Build history of the part. All positions in model axes, mm. A direction names the side the tool comes from. Give positions to 0.01 mm unless a question says otherwise; leave off trailing zeros. Order: outer loops, then holes, each group sorted by start corner. A loop starts at its lowest first (then second) coordinate and runs counter-clockwise, first axis right, second up. Notation, with made-up numbers: (-1.5, 57) - (26.5, 57) arc R21 cw to (26.5, 91) - close; hole circle Ø10 at (22, -12). An arc over 180 degrees is marked (long way). Write each question's results on one line, items separated by ' | '. Start each with the question number.
from build123d import *

# Parameters (mm, degrees)
SKETCH_1_R          = 9
SKETCH_1_R_2        = 2.5
EXTRUDE_1_DEPTH     = 1.5
SKETCH_2_R          = 2.5
EXTRUDE_2_DEPTH     = 7.5
SKETCH_3_R          = 9
SKETCH_3_R_2        = 2.5
EXTRUDE_3_DEPTH     = 9
CHAMFER_2_SIZE      = 0.2
SKETCH_4_R          = 1.75
CUT_EXTRUDE_1_DEPTH = 10
SKETCH_5_R          = 1.75
CUT_EXTRUDE_2_DEPTH = 10


with BuildPart() as part:
    # 草图1 → 凸台-拉伸1 (new body)
    with BuildSketch(Plane.XY):
        Circle(SKETCH_1_R)
        Circle(SKETCH_1_R_2, mode=Mode.SUBTRACT)
    extrude(amount=EXTRUDE_1_DEPTH)

    # 草图2 → 凸台-拉伸2 (add)
    with BuildSketch(Plane.XY.offset(1.5)):
        with BuildLine():
            Line((-0.415, 5.98563071), (-0.415, 4.982747736))
            ThreePointArc((-0.415, 4.982747736), (-0.782172325, 4.938441703), (-1.145065275, 4.867116756))
            Line((-1.145065275, 4.867116756), (-1.454973157, 5.820915144))
            Line((-1.454973157, 5.820915144), (-2.244350066, 5.564431038))
            Line((-2.244350066, 5.564431038), (-1.934442183, 4.610632651))
            ThreePointArc((-1.934442183, 4.610632651), (-2.269952499, 4.455032621), (-2.593043582, 4.275058477))
            Line((-2.593043582, 4.275058477), (-3.182523405, 5.086407846))
            Line((-3.182523405, 5.086407846), (-3.85400751, 4.598546087))
            Line((-3.85400751, 4.598546087), (-3.264527688, 3.787196717))
            ThreePointArc((-3.264527688, 3.787196717), (-3.535533906, 3.535533906), (-3.787196717, 3.264527688))
            Line((-3.787196717, 3.264527688), (-4.598546087, 3.85400751))
            Line((-4.598546087, 3.85400751), (-5.086407846, 3.182523405))
            Line((-5.086407846, 3.182523405), (-4.275058477, 2.593043582))
            ThreePointArc((-4.275058477, 2.593043582), (-4.455032621, 2.269952499), (-4.610632651, 1.934442183))
            Line((-4.610632651, 1.934442183), (-5.564431038, 2.244350066))
            Line((-5.564431038, 2.244350066), (-5.820915144, 1.454973157))
            Line((-5.820915144, 1.454973157), (-4.867116756, 1.145065275))
            ThreePointArc((-4.867116756, 1.145065275), (-4.938441703, 0.782172325), (-4.982747736, 0.415))
            Line((-4.982747736, 0.415), (-5.98563071, 0.415))
            Line((-5.98563071, 0.415), (-5.98563071, -0.415))
            Line((-5.98563071, -0.415), (-4.982747736, -0.415))
            ThreePointArc((-4.982747736, -0.415), (-4.938441703, -0.782172325), (-4.867116756, -1.145065275))
            Line((-4.867116756, -1.145065275), (-5.820915144, -1.454973157))
            Line((-5.820915144, -1.454973157), (-5.564431038, -2.244350066))
            Line((-5.564431038, -2.244350066), (-4.610632651, -1.934442183))
            ThreePointArc((-4.610632651, -1.934442183), (-4.455032621, -2.269952499), (-4.275058477, -2.593043582))
            Line((-4.275058477, -2.593043582), (-5.086407846, -3.182523405))
            Line((-5.086407846, -3.182523405), (-4.598546087, -3.85400751))
            Line((-4.598546087, -3.85400751), (-3.787196717, -3.264527688))
            ThreePointArc((-3.787196717, -3.264527688), (-3.535533906, -3.535533906), (-3.264527688, -3.787196717))
            Line((-3.264527688, -3.787196717), (-3.85400751, -4.598546087))
            Line((-3.85400751, -4.598546087), (-3.182523405, -5.086407846))
            Line((-3.182523405, -5.086407846), (-2.593043582, -4.275058477))
            ThreePointArc((-2.593043582, -4.275058477), (-2.269952499, -4.455032621), (-1.934442183, -4.610632651))
            Line((-1.934442183, -4.610632651), (-2.244350066, -5.564431038))
            Line((-2.244350066, -5.564431038), (-1.454973157, -5.820915144))
            Line((-1.454973157, -5.820915144), (-1.145065275, -4.867116756))
            ThreePointArc((-1.145065275, -4.867116756), (-0.782172325, -4.938441703), (-0.415, -4.982747736))
            Line((-0.415, -4.982747736), (-0.415, -5.98563071))
            Line((-0.415, -5.98563071), (0.415, -5.98563071))
            Line((0.415, -5.98563071), (0.415, -4.982747736))
            ThreePointArc((0.415, -4.982747736), (0.782172325, -4.938441703), (1.145065275, -4.867116756))
            Line((1.145065275, -4.867116756), (1.454973157, -5.820915144))
            Line((1.454973157, -5.820915144), (2.244350066, -5.564431038))
            Line((2.244350066, -5.564431038), (1.934442183, -4.610632651))
            ThreePointArc((1.934442183, -4.610632651), (2.269952499, -4.455032621), (2.593043582, -4.275058477))
            Line((2.593043582, -4.275058477), (3.182523405, -5.086407846))
            Line((3.182523405, -5.086407846), (3.85400751, -4.598546087))
            Line((3.85400751, -4.598546087), (3.264527688, -3.787196717))
            ThreePointArc((3.264527688, -3.787196717), (3.535533906, -3.535533906), (3.787196717, -3.264527688))
            Line((3.787196717, -3.264527688), (4.598546087, -3.85400751))
            Line((4.598546087, -3.85400751), (5.086407846, -3.182523405))
            Line((5.086407846, -3.182523405), (4.275058477, -2.593043582))
            ThreePointArc((4.275058477, -2.593043582), (4.455032621, -2.269952499), (4.610632651, -1.934442183))
            Line((4.610632651, -1.934442183), (5.564431038, -2.244350066))
            Line((5.564431038, -2.244350066), (5.820915144, -1.454973157))
            Line((5.820915144, -1.454973157), (4.867116756, -1.145065275))
            ThreePointArc((4.867116756, -1.145065275), (4.938441703, -0.782172325), (4.982747736, -0.415))
            Line((4.982747736, -0.415), (5.98563071, -0.415))
            Line((5.98563071, -0.415), (5.98563071, 0.415))
            Line((5.98563071, 0.415), (4.982747736, 0.415))
            ThreePointArc((4.982747736, 0.415), (4.938441703, 0.782172325), (4.867116756, 1.145065275))
            Line((4.867116756, 1.145065275), (5.820915144, 1.454973157))
            Line((5.820915144, 1.454973157), (5.564431038, 2.244350066))
            Line((5.564431038, 2.244350066), (4.610632651, 1.934442183))
            ThreePointArc((4.610632651, 1.934442183), (4.455032621, 2.269952499), (4.275058477, 2.593043582))
            Line((4.275058477, 2.593043582), (5.086407846, 3.182523405))
            Line((5.086407846, 3.182523405), (4.598546087, 3.85400751))
            Line((4.598546087, 3.85400751), (3.787196717, 3.264527688))
            ThreePointArc((3.787196717, 3.264527688), (3.535533906, 3.535533906), (3.264527688, 3.787196717))
            Line((3.264527688, 3.787196717), (3.85400751, 4.598546087))
            Line((3.85400751, 4.598546087), (3.182523405, 5.086407846))
            Line((3.182523405, 5.086407846), (2.593043582, 4.275058477))
            ThreePointArc((2.593043582, 4.275058477), (2.269952499, 4.455032621), (1.934442183, 4.610632651))
            Line((1.934442183, 4.610632651), (2.244350066, 5.564431038))
            Line((2.244350066, 5.564431038), (1.454973157, 5.820915144))
            Line((1.454973157, 5.820915144), (1.145065275, 4.867116756))
            ThreePointArc((1.145065275, 4.867116756), (0.782172325, 4.938441703), (0.415, 4.982747736))
            Line((0.415, 4.982747736), (0.415, 5.98563071))
            Line((0.415, 5.98563071), (-0.415, 5.98563071))
        make_face()
        Circle(SKETCH_2_R, mode=Mode.SUBTRACT)
    extrude(amount=EXTRUDE_2_DEPTH)

    # 草图3 → 凸台-拉伸3 (add)
    with BuildSketch(Plane.XY.offset(9)):
        Circle(SKETCH_3_R)
        Circle(SKETCH_3_R_2, mode=Mode.SUBTRACT)
    extrude(amount=EXTRUDE_3_DEPTH)

    # 倒角2
    chamfer_2_edges = [part.edges().sort_by_distance(p)[0] for p in [
        (-9, 0, 0),
        (-9, 0, 18),
        (-9, 0, 9),
        (-2.5, 0, 18),
        (-9, 0, 1.5),
        (-2.5, 0, 0),
    ]]
    chamfer(chamfer_2_edges, length=CHAMFER_2_SIZE)

    # 草图4 → 切除-拉伸1 (cut)
    with BuildSketch(Plane(origin=(0, 0, 0), x_dir=(1, 0, 0), z_dir=(0, 1, 0))):
        with Locations(Location((0, -13.5, 0), (0, 0, 270))):
            Circle(SKETCH_4_R)
    extrude(amount=-CUT_EXTRUDE_1_DEPTH, mode=Mode.SUBTRACT)

    # 草图5 → 切除-拉伸2 (cut)
    with BuildSketch(Plane(origin=(0, 0, 0), x_dir=(0, 0, -1), z_dir=(1, 0, 0))):
        with Locations(Location((-13.5, 0, 0), (0, 0, 180))):
            Circle(SKETCH_5_R)
    extrude(amount=-CUT_EXTRUDE_2_DEPTH, mode=Mode.SUBTRACT)


solid = part.part
Item 1: Two-plate mould, pull along Y, no slides. Class faces 4 (the flat face through (-3.563, 4.199, 5.198)), 5 (the flat face through (5.986, 0, 5)), 6 (the flat face through (2.9, -4.7, 5.2)): +Y half, -Y half, draft (parallel to the pull), parting line (faces both ways), or undercut.
Item 2: Cut at A-A, the plane y = 0. Count the separate pieces of the cut face and the enclosed holes in it, then the cut area to 3 significant figures.
Item 3: Flat gauge pins, fed straight in: pin 1 Ø8 at (x, y) = (0, 0) entering from +Z; pin 2 Ø0.9 at (x, z) = (0, 4) entering from -Y; pin 3 Ø1.1 at (y, z) = (5.5, 6) entering from -X; pin 4 Ø3 at (y, z) = (3.5, 2.5) entering from +X. Where does each tip first touch, or does it go through?
Item 4: Cut at D-D, the plane z = 10.5. List the corners of the cut face in (x, y).
Item 5: Which spindle directions (+Z, -Z, +X, -X, +Y, -Y) get a long thin tool onto all of the face, cutting with end or side? Do faces 1 (the flat face through (4, -4, 9)), 2 (the flat face through (5.35, -1.3, 5.2)), 3 (the flat face through (-5.5, -0.415, 5.2)). Say none if no direction does.
Item 6: Cut at C-C, the plane z = 13.5. List the corners of the cut face in (x, y), then the cut area to 3 significant figures.
Item 7: Probe line 1 along Z through (x, y) = (0, -6.5); line 2 along X through (y, z) = (0, 5); line 3 along Z through (x, y) = (-5, -6). List the from-to ranges inside material, lowest first. Write a range as from..to.
Values found:
1) face 4: undercut | face 5: draft | face 6: -Y half
2) separate pieces: 3 | enclosed holes: 0 | area: 166 mm2
3) pin 1: stops at z = 18 | pin 2: stops at y = -5.99 | pin 3: stops at x = -3.37 | pin 4: stops at x = 8.62
4) outline: circle Ø18 at (0, 0); hole circle Ø5 at (0, 0)
5) face 1: none | face 2: +X | face 3: -X
6) outline: (-8.83, -1.75) arc R9 ccw to (-1.75, -8.83) - (-1.75, -1.79) arc R2.5 cw to (-1.79, -1.75) - close; (-8.83, 1.75) - (-1.79, 1.75) arc R2.5 cw (long way) to (1.75, -1.79) - (1.75, -8.83) arc R9 ccw (long way) to start | area: 188 mm2
7) line 1: z = 0..1.5, 9..11.75, 15.25..18 | line 2: x = -5.99..-2.5, 2.5..5.99 | line 3: z = 0..1.5, 9..18
